Check sheet for the drawn part. Datum: minimum x, y, z corner. Units: mm. Round coordinates to 2 decimals unless told otherwise and drop trailing zeros. Loops run counter-clockwise (first coordinate to the right, second up) from the corner with the lowest first, then second, coordinate; pieces in that order, holes last. Notation, with made-up numbers: (77.5, 55) -> (101.5, 55) arc R37 cw to (101.5, 94) -> close; hole circle Ø2 at (78, 34). An arc over 180 degrees is marked (long way). Return JSON: item names as keys, results as strings.
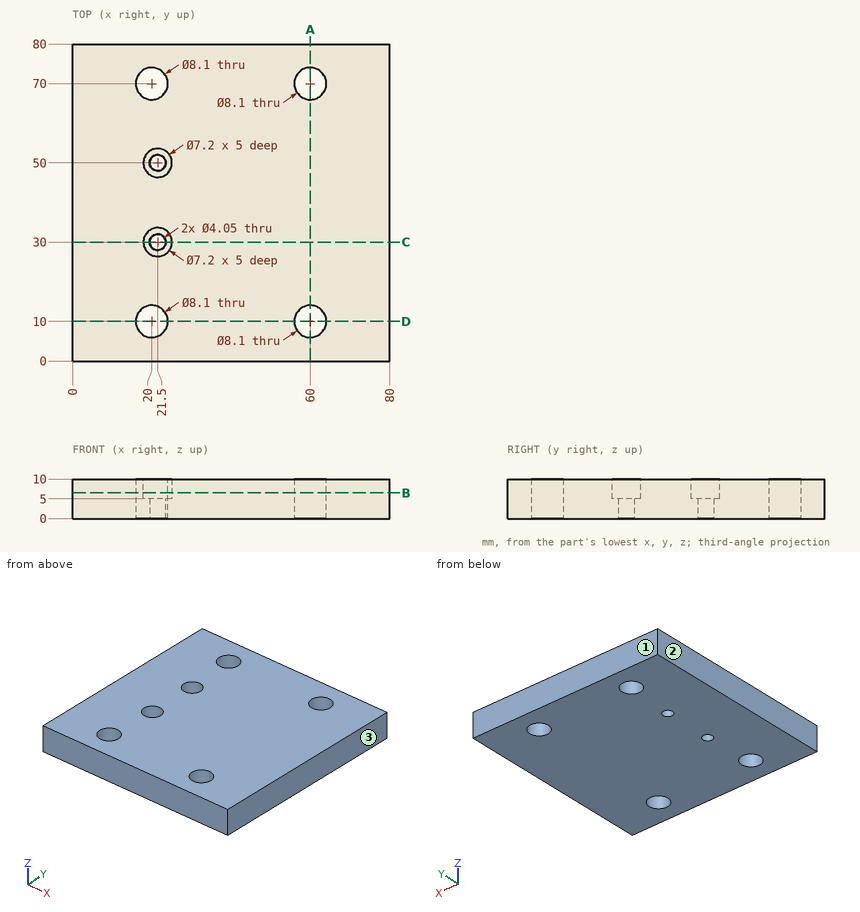
Q1. Go/stop test with flat-tipped pins: pin 1 (3.5 mm diameter, centred on x = 23, y = 49, fed in from +Z); pin 2 (3 mm diameter, centred on x = 21.5, y = 50, fed in from +Z). Record where each tip stops, or that it passes through.
Results list:
{"pin 1": "z = 5", "pin 2": "through"}
Q2. Material ranges on line 1 (Y direction, x = 60, z = 2.25); line 2 (Y direction, x = 21.5, z = 8.6); line 3 (Y direction, x = 16.5, z = 1), recorded low to high.
Results list:
{"line 1": "0 to 5.95, 14.05 to 65.95, 74.05 to 80", "line 2": "0 to 6.24, 13.76 to 26.4, 33.6 to 46.4, 53.6 to 66.24, 73.76 to 80", "line 3": "0 to 7.96, 12.04 to 67.96, 72.04 to 80"}
Q3. Draft check along X on the marked faces 1, 2 and 3. Enter one of: released by +X, released by -X, zero draft, split by the parting line, or undercut.
Results list:
{"face 1": "zero draft", "face 2": "released by -X", "face 3": "released by +X"}
Q4. Section check A-A (x = 60). Record the boundary of the cut face in (y, z), then the cut area to 3 significant figures.
Results list:
{"outline": "(0, 0) -> (5.95, 0) -> (5.95, 10) -> (0, 10) -> close; (14.05, 0) -> (65.95, 0) -> (65.95, 10) -> (14.05, 10) -> close; (74.05, 0) -> (80, 0) -> (80, 10) -> (74.05, 10) -> close", "area": "638 mm^2"}
Q5. Section check B-B (z = 6.5). Record the boundary of the cut face in (x, y), then the cut area to 3 significant figures.
Results list:
{"outline": "(0, 0) -> (80, 0) -> (80, 80) -> (0, 80) -> close; hole circle Ø8.1 at (20, 10); hole circle Ø8.1 at (20, 70); hole circle Ø7.2 at (21.5, 30); hole circle Ø7.2 at (21.5, 50); hole circle Ø8.1 at (60, 10); hole circle Ø8.1 at (60, 70)", "area": "6,110 mm^2"}
Q6. Section check D-D (y = 10). Record the boundary of the cut face in (x, z), then the cut area to 3 significant figures.
Results list:
{"outline": "(0, 0) -> (15.95, 0) -> (15.95, 10) -> (0, 10) -> close; (24.05, 0) -> (55.95, 0) -> (55.95, 10) -> (24.05, 10) -> close; (64.05, 0) -> (80, 0) -> (80, 10) -> (64.05, 10) -> close", "area": "638 mm^2"}
Q7. Section check C-C (y = 30). Record the boundary of the cut face in (x, z) (3 decimals), then the cut area to 3 significant figures.
Results list:
{"outline": "(0, 0) -> (19.475, 0) -> (19.475, 5) -> (17.9, 5) -> (17.9, 10) -> (0, 10) -> close; (23.525, 0) -> (80, 0) -> (80, 10) -> (25.1, 10) -> (25.1, 5) -> (23.525, 5) -> close", "area": "744 mm^2"}
